For this review, take the finished solid that the model builds, in its own axes (mm). Give positions to 0.01 mm unless a question says otherwise; leave off trailing zeros. Loops run counter-clockwise (first coordinate to the right, second up) from the corner with the lowest first, then second, coordinate; pieces in that order, holes last. Notation, with made-up numbers: (79, 6.25) - (110, 6.25) arc R13 cw to (110, 14.25) - close; hole circle Ø4 at (-22, 54.25). An arc over 180 degrees is marked (long way). Use CSV: the item, a comma, the result in double quotes. Start each with the question number.
1. Take a section at C-C on y = 145.5. Give the boundary of the cut face in (x, z), plus the area to 3 significant figures.
2. For pin 1 (5 mm diameter, centred on y = 125, z = 9, fed in from -X); pin 2 (6 mm diameter, centred on x = -61, z = 5, fed in from -Y); pin 3 (10 mm diameter, centred on x = 11, y = 51, fed in from -Z); pin 4 (3 mm diameter, centred on y = 143.5, z = 4.5, fed in from -X), all flat-tipped, find the tip position at first contact; note any pin that passes through.
3. Take a section at D-D on y = 61. Give the boundary of the cut face in (x, z), plus the area to 3 significant figures.
4. Wall thickness on line 1 (Y direction, x = -90, z = 4.25); line 2 (Y direction, x = -50, z = 7.25); line 3 (X direction, y = 80.5, z = 1): over which ranges is each line inside the solid? List them lowest first.
5. Take a section at A-A on z = 4.5. State how many separate pieces and enclosed holes the cut face has, plus the area to 3 significant figures.
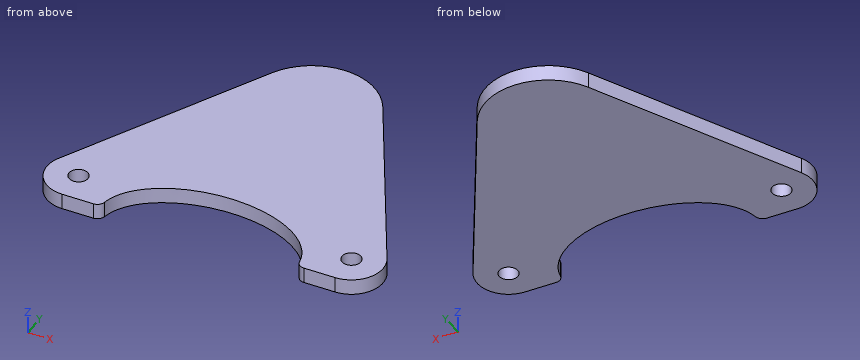
```python
from build123d import *

# Parameters (mm, degrees)
F1_DEPTH = 10
F3_D     = 12
F5_DEPTH = 25
F6_R     = 5


# Not quite as in the source:
# - a pattern or mirror of a feature is missing from the dataset's text; its kind, count and spacing are read off the source's solid


with BuildPart() as f1:
    # F0 (on Top) → F1 (new body)
    with BuildSketch(Plane.XY):
        with BuildLine():
            Line((-86.4857615178, 0), (0, 0))
            Line((0, 0), (86.4857615178, 0))
            ThreePointArc((86.4857615178, 0), (103.6601107493, 9.7510132951), (104.0877292116, 29.4958271523))
            Line((104.0877292116, 29.4958271523), (35.2039353876, 157.1824724621))
            ThreePointArc((35.2039353876, 157.1824724621), (0, 178.1908181575), (-35.2039353876, 157.1824724621))
            Line((-35.2039353876, 157.1824724621), (-104.0877292116, 29.4958271523))
            ThreePointArc((-104.0877292116, 29.4958271523), (-103.6601107493, 9.7510132951), (-86.4857615178, 0))
        make_face()
    extrude(amount=F1_DEPTH)

    # F3 (through all)
    with Locations(Plane.XY.offset(10)):
        with Locations((86.4857615178, 20)):
            f3 = Hole(F3_D / 2)

    # F3_copies: F3 across plane
    add(f3.mirror(Plane(origin=(0, 0, 0), x_dir=(0, 0, -1), z_dir=(-1, 0, 0))), mode=Mode.SUBTRACT)

    # F4 (on face) → F5 (cut)
    with BuildSketch(Plane.XY.offset(10)):
        with BuildLine():
            add(Edge.make_bspline(
                [(62.1145702899, 0), (62.1145702899, 69.1070951712), (-31.0572851449, 34.5535475856), (-124.2291405797, 0), (-31.0572851449, -34.5535475856), (62.1145702899, -69.1070951712), (62.1145702899, 0)],
                knots=[0, 0, 0, 2.0943951024, 2.0943951024, 4.1887902048, 4.1887902048, 6.2831853072, 6.2831853072, 6.2831853072], degree=2, weights=[1, 0.5, 1, 0.5, 1, 0.5, 1]))
        make_face()
    extrude(amount=-F5_DEPTH, mode=Mode.SUBTRACT)

    # F6
    f6_edges = [f1.edges().sort_by_distance(p)[0] for p in [
        (-62.11457, 0, 5),
        (62.11457, 0, 5),
    ]]
    fillet(f6_edges, radius=F6_R)


solid = f1.part
```
Check result:
1,outline,"(-41.51, 0) - (41.51, 0) - (41.51, 10) - (-41.51, 10) - close"
1,area,"830 mm²"
2,pin 1,"stops at x = -53.91"
2,pin 2,"stops at y = 0.79"
2,pin 3,"stops at z = 0"
2,pin 4,"stops at x = -43.39"
3,outline,"(-87.09, 0) - (87.09, 0) - (87.09, 10) - (-87.09, 10) - close"
3,area,"1,740 mm²"
4,line 1,"y = 0.31 to 15.14, 24.86 to 55.61"
4,line 2,"y = 23.67 to 129.76"
4,line 3,"x = -76.57 to 76.57"
5,separate pieces,"1"
5,enclosed holes,"2"
5,area,"20,800 mm²"
